Verification items for the finished model (mm, model axes). A direction names the side the tool comes from. Give positions to 0.01 mm unless a question says otherwise; leave off trailing zeros. Write each loop counter-clockwise with the first axis right and the second up, starting at its lowest first coordinate (ties: lowest second). Pieces come first, ordered by that corner, then holes. Notation, with made-up numbers: (-9.75, -21.5) -> (22.25, -21.5) arc R16 ccw to (22.25, 3.5) -> close; hole circle Ø6 at (6.25, 58.5). An arc over 180 degrees is marked (long way). Answer as CSV lines item,"result". Start each with the question number.
1) Sectioned sample at C-C on x = 12.5. Record the cut outline in (y, z).
2) Tool access check on faces 4 (the flat face through (17.325, 0.986, 11.55)), 5 (the flat face through (15, 1, -15)). Record the directions out of +Z, -Z, +X, -X, +Y, -Y that give a thin tool (end or side, any length) a straight path to the whole face; none if there is none.
3) Gauge pin test, flat ends, axial feed: pin 1 Ø1 at (y, z) = (0.5, 7) entering from -X; pin 2 Ø1 at (x, y) = (24, 1.5) entering from +Z. Record the tip position at first contact, or that the pin passes through.
4) Material ranges on L1, parallel to X at y = 1.35, z = -1; L2, parallel to X at y = 1.45, z = -11, recorded low to high.
5) Sectioned sample at A-A on z = -6.5. Record the cut outline in (x, y).
6) Mould release check, pull along X, two halves, no side actions. Record for faces 1 (the flat face through (15, 1, 15)), 2 (the flat face through (18, 1, -12)), 3 (the flat face through (80, 2, 0)): released by +X, released by -X, zero draft, split by the parting line, or undercut.
7) Sectioned sample at B-B on y = 0.6. Record the cut outline in (x, z).
```python
from build123d import *

# Parameters (mm, degrees)
BOSS_EXTRUDE1_DEPTH = 2


with BuildPart() as part:
    # Sketch1 → Boss-Extrude1 (new body)
    with BuildSketch(Plane(origin=(0, 0, 0), x_dir=(1, 0, 0), z_dir=(0, 1, 0))):
        Polygon((0, 5), (30, 25), (130, 25), (130, -25), (30, -25), (0, -5), align=None)
        Polygon((30, -20), (30, 20), (5, 3.333333333), (5, -3.333333333), align=None, mode=Mode.SUBTRACT)
    extrude(amount=BOSS_EXTRUDE1_DEPTH)


solid = part.part
```
Ans:
1,outline,"(0, -13.33) -> (2, -13.33) -> (2, -8.33) -> (0, -8.33) -> close; (0, 8.33) -> (2, 8.33) -> (2, 13.33) -> (0, 13.33) -> close"
2,face 4,"+Y, -Y"
2,face 5,"-Z, -X, +Y, -Y"
3,pin 1,"stops at x = 2.25"
3,pin 2,"stops at z = 21.33"
4,L1,"x = 0 to 5, 30 to 130"
4,L2,"x = 9 to 16.5, 30 to 130"
5,outline,"(2.25, 0) -> (9.75, 0) -> (9.75, 2) -> (2.25, 2) -> close; (30, 0) -> (130, 0) -> (130, 2) -> (30, 2) -> close"
6,face 1,"released by -X"
6,face 2,"undercut"
6,face 3,"zero draft"
7,outline,"(0, -5) -> (30, -25) -> (130, -25) -> (130, 25) -> (30, 25) -> (0, 5) -> close; hole (5, -3.33) -> (30, -20) -> (30, 20) -> (5, 3.33) -> close"
